CAD build for the part. Positions are in the model's coordinates, mm. Face numbers are marked on the shaded views. A direction names the side the tool comes from. Give positions to 0.01 mm unless a question says otherwise; leave off trailing zeros. Order: outer loops, then holes, each group sorted by start corner. A loop starts at its lowest first (then second) coordinate and runs counter-clockwise, first axis right, second up. Notation, with made-up numbers: (-5, 83) -> (32, 83) arc R27 ccw to (32, 99) -> close; hole circle Ø2 at (-7.75, 9). An arc over 180 degrees is marked (long way). Use one line per item in the form item = value. Start each with the question number.
1) Cut at C-C, the plane z = 18.75. Give the cut face in (x, y), and give its area (3 significant figures).
2) Mould opens along Y. For the marked faces 1, 2 and 3 say: pulls with the +Y half, pulls with the -Y half, needs draft (parallel to the pull), parting line crosses it, or undercut.
3) Probe line 1 (Y direction, x = 96, z = 14); line 2 (Z direction, x = 78.5, y = 0.8); line 3 (Z direction, x = 136.5, y = 17). List the from-to ranges inside material, lowest first.
4) Cut at B-B, the plane x = 121. Give the cut face in (y, z), and give its area (3 significant figures).
5) Cut at D-D, the plane z = 8. Give the cut face in (x, y).
6) Drop flat-ended pins along their axis: P1, Ø2, axis at x = 141, z = 16, coming from the -Y side; P2, Ø0.7, axis at x = 18.5, z = 23, coming from the -Y side; P3, Ø1.5, axis at x = 127, y = 11, coming from the +Z side; P4, Ø6.5, axis at y = 13, z = 17.5, coming from the +X side. Give the stop position or say it passes through.
7) Tool access for the marked faces 4 and 5: list every direction of +Z, -Z, +X, -X, +Y, -Y with a clear straight run to the whole face (end or side of a thin tool).
8) Cut at A-A, the plane y = 6.5. Give the cut face in (x, z), and give its area (3 significant figures).
from build123d import *

# Parameters (mm, degrees)
CYLINDER003_R     = 2
CYLINDER003_DEPTH = 10
ARRAY001_Y_COUNT  = 2
ARRAY001_Y_PITCH  = 13.5
CYLINDER002_R     = 0.6
CYLINDER002_DEPTH = 100
ARRAY002_X_COUNT  = 8
ARRAY002_X_PITCH  = 20
BOX001_W          = 170
BOX001_H          = 21.76
BOX001_DEPTH      = 26.3
BOX_W             = 170
BOX_H             = 25.76
BOX_DEPTH         = 26.3


with BuildPart() as array001:
    # Cylinder003 → Cylinder003 (new body)
    with BuildSketch(Plane(origin=(-4, 6.5, 19), x_dir=(0, 0, -1), z_dir=(1, 0, 0))):
        Circle(CYLINDER003_R)
    extrude(amount=CYLINDER003_DEPTH)

    # Array001 Y: Array001 ×2


with BuildPart() as array001_1:
    add(array001.part)
    with Locations(*[(0, i * ARRAY001_Y_PITCH, 0) for i in range(1, ARRAY001_Y_COUNT)]):
        add(array001.part)


with BuildPart() as array002:
    # Cylinder002 → Cylinder002 (new body)
    with BuildSketch(Plane(origin=(18.5, -32.5, 23), x_dir=(1, 0, 0), z_dir=(0, 1, 0))):
        Circle(CYLINDER002_R)
    extrude(amount=CYLINDER002_DEPTH)

    # Array002 X: Array002 ×8


with BuildPart() as array002_1:
    add(array002.part)
    with Locations(*[(i * ARRAY002_X_PITCH, 0, 0) for i in range(1, ARRAY002_X_COUNT)]):
        add(array002.part)


with BuildPart() as fusion:
    # Box001 → Box001 (new body)
    with BuildSketch(Plane(origin=(2, 2, 2), x_dir=(1, 0, 0), z_dir=(0, 0, 1))):
        with Locations((85, 10.88)):
            Rectangle(BOX001_W, BOX001_H)
    extrude(amount=BOX001_DEPTH)

    # Fusion: union Array001, Array002
    add(array001_1.part)
    add(array002_1.part)


with BuildPart() as cut001:
    # Box → Box (new body)
    with BuildSketch(Plane.XY):
        with Locations((85, 12.88)):
            Rectangle(BOX_W, BOX_H)
    extrude(amount=BOX_DEPTH)

    # Cut001: cut Fusion
    add(fusion.part, mode=Mode.SUBTRACT)


solid = cut001.part
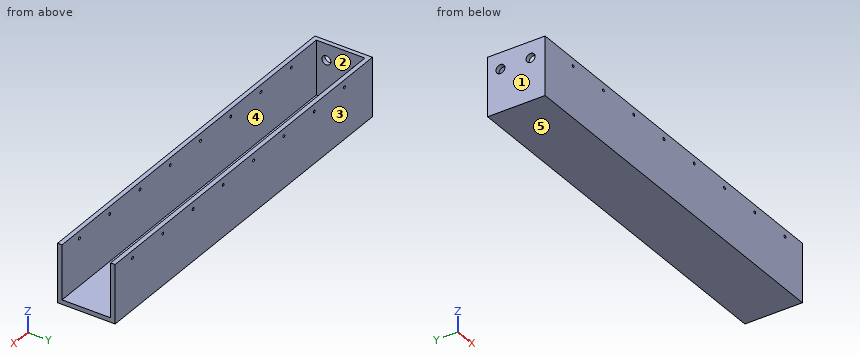
Result:
q1.outline = (0, 0) -> (170, 0) -> (170, 2) -> (2, 2) -> (2, 4.52) -> (0, 4.52) -> close; (0, 8.48) -> (2, 8.48) -> (2, 18.02) -> (0, 18.02) -> close; (0, 21.98) -> (2, 21.98) -> (2, 23.76) -> (170, 23.76) -> (170, 25.76) -> (0, 25.76) -> close
q1.area = 708 mm²
q2.face_1 = needs draft
q2.face_2 = undercut
q2.face_3 = pulls with the +Y half
q3.line_1 = 0 to 2, 23.76 to 25.76
q3.line_2 = 0 to 22.4, 23.6 to 26.3
q3.line_3 = 0 to 2
q4.outline = (0, 0) -> (25.76, 0) -> (25.76, 26.3) -> (23.76, 26.3) -> (23.76, 2) -> (2, 2) -> (2, 26.3) -> (0, 26.3) -> close
q4.area = 149 mm²
q5.outline = (0, 0) -> (170, 0) -> (170, 2) -> (2, 2) -> (2, 23.76) -> (170, 23.76) -> (170, 25.76) -> (0, 25.76) -> close
q6.P1 = 0
q6.P2 = through
q6.P3 = 2
q6.P4 = 2
q7.face_4 = +Z, +X
q7.face_5 = -Z, +X, -X, +Y, -Y
q8.outline = (0, 0) -> (170, 0) -> (170, 2) -> (2, 2) -> (2, 17) -> (0, 17) -> close; (0, 21) -> (2, 21) -> (2, 26.3) -> (0, 26.3) -> close
q8.area = 381 mm²
